Autodesk Inventor part; units mm, degrees
ref_plane "YZ Plane" through (0, 0, 0) normal (1, 0, 0) x (0, 1, 0)
ref_plane "XZ Plane" through (0, 0, 0) normal (0, 1, 0) x (-1, 0, 0)
ref_plane "XY Plane" through (0, 0, 0) normal (0, 0, 1) x (1, 0, 0)
sketch "Sketch1" plane through (0, 0, 0) normal (1, 0, 0) x (0, 1, 0)
  line L0 (5, -17.593) -> (-5, -17.593)
  line L1 (-5, -17.593) -> (-5, 17.593)
  line L2 (-5, 17.593) -> (5, 17.593)
  line L3 (5, 17.593) -> (5, -17.593)
  line L4 (5, -17.593) -> (-5, 17.593) construction
  line L5 (-5, -17.593) -> (5, 17.593) construction
  point P0 (0, 0)
  dimension "d0" = 35.186
  dimension "d2" = 10
extrude "Extrusion1" add sketch "Sketch1" along normal blind 2
sketch "Sketch2" plane through (2, 0, 0) normal (1, 0, 0) x (0, 0, -1)
  circle A0 centre (0, 0) radius 4
  dimension "d5" = 8
extrude "Extrusion2" add sketch "Sketch2" along normal blind 5
sketch "Sketch3" plane through (7, 0, 0) normal (1, 0, 0) x (0, 0, -1)
  circle A0 centre (0, 0) radius 4
  circle A1 centre (0, 0) radius 2
  dimension "d8" = 4
extrude "Extrusion3" cut sketch "Sketch3" against normal blind 7 contours A1
sketch "Sketch4" plane through (2, 0, 0) normal (1, 0, 0) x (0, 0, -1)
  line L0 (-17.593, 5) -> (-12.593, 5)
  line L1 (-12.593, 5) -> (-12.593, 0)
  line L2 (-12.593, 0) -> (-17.593, 0)
  line L3 (-17.593, 0) -> (-17.593, 5)
  line L4 (17.593, 5) -> (12.593, 5)
  line L5 (12.593, 5) -> (12.593, 0)
  line L6 (12.593, 0) -> (17.593, 0)
  line L7 (17.593, 0) -> (17.593, 5)
  circle A0 centre (-12.593, 0) radius 1.5
  circle A1 centre (12.593, 0) radius 1.5
  dimension "d11" = 5
  dimension "d12" = 5
  dimension "d13" = 3
  dimension "d14" = 3
extrude "Extrusion4" cut sketch "Sketch4" against normal blind 2 contours A0 L2 L1 | L1 L2 A0 | A1 L6 L5 | L5 L6 A1
chamfer "Chamfer1" distance 1 angle 45 1 edges at (7, 0, 4)
chamfer "Chamfer2" distance 2 angle 45 2 edges at (2, 0, -17.593) (2, 0, 17.593)
properties part number "paka_packa" material "Iron, Cast"
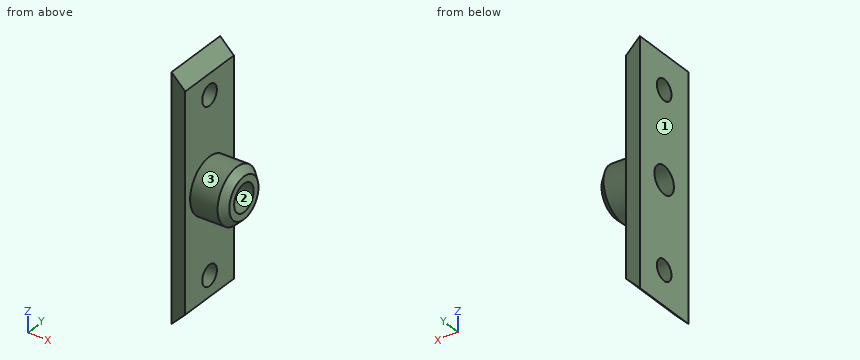
Model file for the job. Use its own axes, mm. Face numbers are marked on the shaded views. Give positions to 0.01 mm unless a question says otherwise; leave off trailing zeros. Order: outer loops, then holes, each group sorted by start corner. A loop starts at its lowest first (then second) coordinate and runs counter-clockwise, first axis right, second up. Notation, with made-up numbers: (-20, 88.25) -> (-1, 88.25) arc R7 ccw to (-1, 94.25) -> close; hole circle Ø10 at (-36, -31). An arc over 180 degrees is marked (long way). Use CSV: the item, a comma, the result in double quotes.
1. Band-saw the part on B-B, the plane y = 0. Count the separate pieces of the cut face and the enclosed holes in it, then the cut area to 3 significant figures.
Outcome:
separate pieces,"4"
enclosed holes,"0"
area,"65.4 mm²"
2. Mould opens along Y. For the marked faces 1, 2 and 3 say: +Y half, -Y half, draft (parallel to the pull), parting line (faces both ways), or undercut.
Outcome:
face 1,"draft"
face 2,"undercut"
face 3,"parting line"
3. Drill centre lines: line 1 along X through (y, z) = (0.25, -5); line 2 along Y through (x, z) = (2.75, 0); line 3 along Z through (x, y) = (2.5, 0.25). Where is each one in solid material? Low to high. Write a range as from..to.
Outcome:
line 1,"0..2"
line 2,"-4..-2, 2..4"
line 3,"-3.99..-1.98, 1.98..3.99"
4. Band-saw the part on A-A, the plane z = 0. Give the cut face in (x, y).
Outcome:
outline,"(0, -5) -> (2, -5) -> (2, -4) -> (6, -4) -> (7, -3) -> (7, -2) -> (0, -2) -> close; (0, 2) -> (7, 2) -> (7, 3) -> (6, 4) -> (2, 4) -> (2, 5) -> (0, 5) -> close"
5. Drop flat-ended pins along their axis: pin 1 (4 mm diameter, centred on x = 1.5, y = 4, fed in from +Z); pin 2 (4 mm diameter, centred on y = 0, z = -12.593, fed in from +X); pin 3 (2 mm diameter, centred on x = 3.5, y = 2.5, fed in from +Z). Give the stop position or say it passes through.
Outcome:
pin 1,"z = 17.59"
pin 2,"x = 2"
pin 3,"z = 3.71"
6. Band-saw the part on D-D, the plane x = 1.5. Give the cut face in (y, z), then the cut area to 3 significant figures.
Outcome:
outline,"(-5, -16.09) -> (5, -16.09) -> (5, 16.09) -> (-5, 16.09) -> close; hole circle Ø4 at (0, 0); hole circle Ø3 at (0, -12.59); hole circle Ø3 at (0, 12.59)"
area,"295 mm²"
7. Band-saw the part on C-C, the plane x = 3. Give the cut face in (y, z), then the cut area to 3 significant figures.
Outcome:
outline,"circle Ø8 at (0, 0); hole circle Ø4 at (0, 0)"
area,"37.7 mm²"
